Check sheet for the modelled part. Datum: model origin and axes. Units: mm. A direction names the side the tool comes from. Coordinates: 2 decimals unless noted, no trailing zeros. Loops run counter-clockwise (first coordinate to the right, second up) from the corner with the lowest first, then second, coordinate; pieces in that order, holes last. Notation, with made-up numbers: M 14,17 L 65,17 A28 cw 65,40 Z; hole C 16.25,72 d9. An arc over 180 degrees is marked long. Answer in a Markdown table with one row per item. Add a question column.
```python
from build123d import *

# Parameters (mm, degrees)
F1_DEPTH = 6.35
F2_DEPTH = 12.7
F4_DEPTH = 6.35
F5_SIZE  = 2.54
F3_W     = 8.288401
F3_H     = 6.35
F6_DEPTH = 6.35
F7_SIZE  = 2.54


with BuildPart() as f1:
    # F0 (on Front) → F1 (new body)
    with BuildSketch(Plane.XZ):
        with BuildLine():
            Line((50.8, 31.75), (-50.8, 31.75))
            ThreePointArc((-50.8, 31.75), (-82.55, 0), (-50.8, -31.75))
            Line((-50.8, -31.75), (50.8, -31.75))
            ThreePointArc((50.8, -31.75), (82.55, 0), (50.8, 31.75))
        make_face()
        with BuildLine():
            ThreePointArc((-50.6538152695, -3.175), (-53.8288152695, 0), (-50.6538152695, 3.175))
            Line((-50.6538152695, 3.175), (50.6538152695, 3.175))
            ThreePointArc((50.6538152695, 3.175), (53.8288152695, 0), (50.6538152695, -3.175))
            Line((50.6538152695, -3.175), (-50.6538152695, -3.175))
        make_face(mode=Mode.SUBTRACT)
    extrude(amount=F1_DEPTH)

    # F0 (on Front) → F2 (join)
    with BuildSketch(Plane.XZ):
        with BuildLine():
            Line((50.8, 38.1), (-50.8, 38.1))
            ThreePointArc((-50.8, 38.1), (-88.9, 0), (-50.8, -38.1))
            Line((-50.8, -38.1), (50.8, -38.1))
            ThreePointArc((50.8, -38.1), (88.9, 0), (50.8, 38.1))
        make_face()
        with BuildLine():
            ThreePointArc((-50.8, -31.75), (-82.55, 0), (-50.8, 31.75))
            Line((-50.8, 31.75), (50.8, 31.75))
            ThreePointArc((50.8, 31.75), (82.55, 0), (50.8, -31.75))
            Line((50.8, -31.75), (-50.8, -31.75))
        make_face(mode=Mode.SUBTRACT)
    extrude(amount=F2_DEPTH)

    # F3 (on face) → F4 (join)
    with BuildSketch(Plane.XZ.offset(6.35)):
        Polygon((-38.1, -31.75), (-33.9557995, -31.75), (-33.9557995, -25.4), (-38.1, -25.4), (-42.2442005, -25.4), (-42.2442005, -31.75), align=None)
        Polygon((-27.0042005, -31.75), (-18.7157995, -31.75), (-18.7157995, -25.4), (-22.86, -25.4), (-27.0042005, -25.4), align=None)
        Polygon((-11.7515005, -31.75), (-3.4757995, -31.75), (-3.4757995, -25.4), (-7.62, -25.4), (-11.7515005, -25.4), align=None)
        Polygon((3.4757995, -25.4), (3.4757995, -31.75), (11.7642005, -31.75), (11.7642005, -25.4), (7.62, -25.4), align=None)
        Polygon((18.7157995, -25.4), (18.7157995, -31.75), (27.0042005, -31.75), (27.0042005, -25.4), (22.86, -25.4), align=None)
        Polygon((33.9557995, -25.4), (33.9557995, -31.75), (38.1, -31.75), (42.2442005, -31.75), (42.2442005, -25.4), (38.1, -25.4), align=None)
    extrude(amount=F4_DEPTH)

    # F5
    f5_edges = [f1.edges().sort_by_distance(p)[0] for p in [
        (-42.244201, -9.525, -25.4),
        (-33.9558, -9.525, -25.4),
        (-27.004201, -9.525, -25.4),
        (-18.7158, -9.525, -25.4),
        (-11.751501, -9.525, -25.4),
        (-3.4758, -9.525, -25.4),
        (3.475799, -9.525, -25.4),
        (11.7642, -9.525, -25.4),
        (18.715799, -9.525, -25.4),
        (27.0042, -9.525, -25.4),
        (33.9558, -9.525, -25.4),
        (42.244201, -9.525, -25.4),
        (33.9558, -9.525, -31.75),
        (42.244201, -9.525, -31.75),
        (27.0042, -9.525, -31.75),
        (11.7642, -9.525, -31.75),
        (18.715799, -9.525, -31.75),
        (3.475799, -9.525, -31.75),
        (-11.751501, -9.525, -31.75),
        (-27.004201, -9.525, -31.75),
        (-3.4758, -9.525, -31.75),
        (-18.7158, -9.525, -31.75),
        (-33.9558, -9.525, -31.75),
        (-42.244201, -9.525, -31.75),
    ]]
    chamfer(f5_edges, length=F5_SIZE)

    # F3 (on face) → F6 (join)
    with BuildSketch(Plane.XZ.offset(6.35)):
        with Locations((-38.1, 28.575)):
            Rectangle(F3_W, F3_H)
        with Locations((-22.86, 28.575)):
            Rectangle(F3_W, F3_H)
        Polygon((-3.4757995, 31.75), (-11.7515005, 31.75), (-11.7515005, 25.4), (-7.62, 25.4), (-3.4757995, 25.4), align=None)
        Polygon((11.7642005, 25.4), (11.7642005, 31.75), (3.4757995, 31.75), (3.4757995, 25.4), (7.62, 25.4), align=None)
        Polygon((27.0042005, 25.4), (27.0042005, 31.75), (18.7157995, 31.75), (18.7157995, 25.4), (22.86, 25.4), align=None)
        Polygon((42.2442005, 25.4), (42.2442005, 31.75), (33.9557995, 31.75), (33.9557995, 25.4), (38.1, 25.4), align=None)
    extrude(amount=F6_DEPTH)

    # F7
    f7_edges = [f1.edges().sort_by_distance(p)[0] for p in [
        (-42.244201, -9.525, 31.75),
        (-27.004201, -9.525, 31.75),
        (-42.244201, -9.525, 25.4),
        (-33.9558, -9.525, 25.4),
        (-33.955799, -9.525, 31.75),
        (-27.004201, -9.525, 25.4),
        (-18.7158, -9.525, 25.4),
        (-18.7158, -9.525, 31.75),
        (-11.751501, -9.525, 25.4),
        (-11.7515, -9.525, 31.75),
        (-3.4758, -9.525, 25.4),
        (3.475799, -9.525, 25.4),
        (11.7642, -9.525, 25.4),
        (18.715799, -9.525, 25.4),
        (27.0042, -9.525, 25.4),
        (33.9558, -9.525, 25.4),
        (42.244201, -9.525, 25.4),
        (42.244201, -9.525, 31.75),
        (27.0042, -9.525, 31.75),
        (11.764201, -9.525, 31.75),
        (18.7158, -9.525, 31.75),
        (33.9558, -9.525, 31.75),
        (-3.4758, -9.525, 31.75),
        (3.475799, -9.525, 31.75),
    ]]
    chamfer(f7_edges, length=F7_SIZE)


solid = f1.part
```
Q1. Go/stop test with flat-tipped pins: pin 1 (1 mm diameter, centred on y = -9, z = 28.5, fed in from -X); pin 2 (3 mm diameter, centred on y = -7, z = 5, fed in from -X); pin 3 (0.6 mm diameter, centred on y = -8.5, z = 28.5, fed in from -X). Record where each tip stops, or that it passes through.
Q2. Cross-section at D-D (z = 33.5). Record the cut outline in (x, y), plus the area to 3 significant figures.
Q3. Cross-section at C-C (x = -64.5). Record the cut outline in (y, z), plus the area to 3 significant figures.
Q4. Cross-section at B-B (z = -17). Record the cut outline in (x, y).
Q5. Thickness scan on L1, parallel to Z at x = -21, y = -2.75 (3 decimals); L2, parallel to Z at x = -21.5, y = -8; L3, parallel to Y at x = -71, z = 7. Record the ranges inside material, lowest first.
Q6. Cross-section at A-A (z = 0). Record the cut outline in (x, y).
Q7. Access from +Z, -Z, +X, -X, +Y, -Y to the whole of each face (thin tool, end or side, straight path). Record for faces 1 (the face through (88.89, -6.26, -0.84)), 2 (the face through (-1, -3, 3.175)), 3 (the face through (-1, -6.35, -7)).
Answer key:
| question | item | result |
|---|---|---|
| 1 | pin 1 | x = -76.64 |
| 1 | pin 2 | x = -88.74 |
| 1 | pin 3 | x = -76.42 |
| 2 | outline | M -68.95,-12.7 L 68.95,-12.7 L 68.95,0 L -68.95,0 Z |
| 2 | area | 1,750 mm^2 |
| 3 | outline | M -12.7,-35.55 L 0,-35.55 L 0,35.55 L -12.7,35.55 L -12.7,28.64 L -6.35,28.64 L -6.35,-28.64 L -12.7,-28.64 Z |
| 3 | area | 539 mm^2 |
| 4 | outline | M -84.9,-12.7 L -77.62,-12.7 L -77.62,-6.35 L 77.62,-6.35 L 77.62,-12.7 L 84.9,-12.7 L 84.9,0 L -84.9,0 Z |
| 5 | L1 | -38.1 to -3.175, 3.175 to 38.1 |
| 5 | L2 | -38.1 to -25.4, 25.4 to 38.1 |
| 5 | L3 | -6.35 to 0 |
| 6 | outline | M -88.9,-12.7 L -82.55,-12.7 L -82.55,-6.35 L -53.83,-6.35 L -53.83,0 L -88.9,0 Z; M 53.83,-6.35 L 82.55,-6.35 L 82.55,-12.7 L 88.9,-12.7 L 88.9,0 L 53.83,0 Z |
| 7 | face 1 | +X, +Y, -Y |
| 7 | face 2 | +Y, -Y |
| 7 | face 3 | -Y |
